```python
from build123d import *

# Parameters (mm, degrees)
ESBO_O1_R                = 2.5
ESBO_O1_W                = 20
ESBO_O1_H                = 40
RESSALTO_EXTRUS_O1_DEPTH = 20
RESSALTO_EXTRUS_O2_DEPTH = 20


with BuildPart() as part:
    # Esboço1 → Ressalto-extrusão1 (new body)
    with BuildSketch(Plane.XY):
        Polygon((2.323964608, -15.698616601), (-17.676035392, -15.698616601), (-21.676035392, -15.698616601), (-21.676035392, 34.301383399), (-21.676035392, 44.301383399), (6.323964608, 44.301383399), (6.323964608, 34.301383399), (6.323964608, -15.698616601), align=None)
        with Locations((-12.176035392, -9.998616601)):
            Circle(ESBO_O1_R, mode=Mode.SUBTRACT)
        with Locations((-3.176035392, -9.998616601)):
            Circle(ESBO_O1_R, mode=Mode.SUBTRACT)
        with Locations((-12.176035392, 38.601383399)):
            Circle(ESBO_O1_R, mode=Mode.SUBTRACT)
        with Locations((-3.176035392, 38.601383399)):
            Circle(ESBO_O1_R, mode=Mode.SUBTRACT)
        with Locations((-7.676035392, 14.301383399)):
            Rectangle(ESBO_O1_W, ESBO_O1_H, mode=Mode.SUBTRACT)
    extrude(amount=RESSALTO_EXTRUS_O1_DEPTH)

    # Esboço2 → Ressalto-extrusão2 (add)
    with BuildSketch(Plane(origin=(0, 0, 0), x_dir=(-1, 0, 0), z_dir=(0, 0, -1))):
        Polygon((-6.323964608, 44.301383399), (-6.323964608, -15.698616601), (-11.323964608, -15.698616601), (-11.323964608, 96.069751334), (-6.323964608, 96.069751334), align=None)
    extrude(amount=-RESSALTO_EXTRUS_O2_DEPTH)


solid = part.part
```
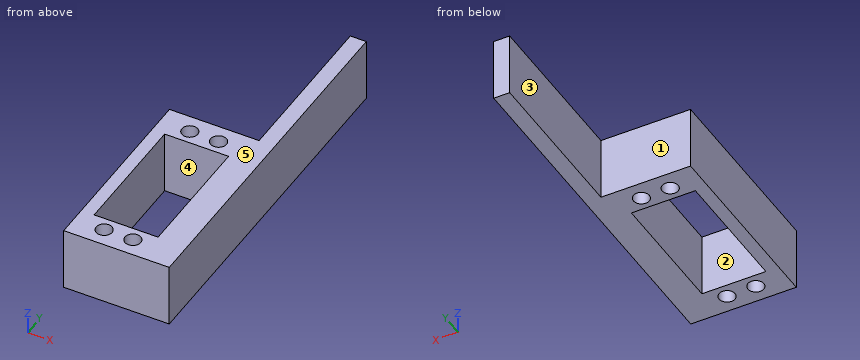
The listing builds one solid part. Answer for the finished solid, in the listing's coordinates (mm). Face numbers are marked on the shaded views. A direction names the side the tool comes from. Coordinates: 2 decimals unless noted, no trailing zeros. Loops run counter-clockwise (first coordinate to the right, second up) from the corner with the lowest first, then second, coordinate; pieces in that order, holes last. Notation, with made-up numbers: (-9.5, 38.25) - (44.5, 38.25) arc R31 cw to (44.5, 74.25) - close; hole circle Ø6 at (84.25, 74.5). An arc over 180 degrees is marked (long way). Write item = value, one per line.
1) Determine the mould class of the marked faces 1, 2 and 3 for opening direction Y: pulls with the +Y half, pulls with the -Y half, needs draft (parallel to the pull), parting line crosses it, or undercut.
Responses:
face_1 = pulls with the +Y half
face_2 = undercut
face_3 = needs draft
2) Which of the six approach directions +Z, -Z, +X, -X, +Y, -Y give full straight-line access (tool end or side, diameter ignored) to the marked faces 4 and 5?
Responses:
face_4 = +Z, -Z
face_5 = +Z, +X, -X, +Y, -Y
3) Find the intervals of material crossed by line 1 along X through (y, z) = (4.5, 18.25); line 2 along Y through (x, z) = (-6.5, 17.25); line 3 along Y through (x, z) = (-11, 19), in increasing order.
Responses:
line_1 = -21.68 to -17.68, 2.32 to 11.32
line_2 = -15.7 to -5.7, 34.3 to 44.3
line_3 = -15.7 to -12.2, -7.79 to -5.7, 34.3 to 36.4, 40.81 to 44.3
4) Section D-D (x = 4) is taken. Determine the outline of the cut face in (y, z).
Responses:
outline = (-15.7, 0) - (44.3, 0) - (44.3, 20) - (-15.7, 20) - close
5) Each of these flat-tipped pins is pushed along its axis until it touches: P1, Ø8, axis at x = -8, z = 4, coming from the +Y side; P2, Ø3, axis at x = -12.18, y = 38.6, coming from the -Z side; P3, Ø2, axis at y = 68.5, z = 3.5, coming from the -X side. Where does it stop, or does it pass through?
Responses:
P1 = 44.3
P2 = through
P3 = 6.32
6) Section C-C (z = 1.5) is taken. Determine the outline of the cut face in (x, y).
Responses:
outline = (-21.68, -15.7) - (11.32, -15.7) - (11.32, 96.07) - (6.32, 96.07) - (6.32, 44.3) - (-21.68, 44.3) - close; hole (-17.68, -5.7) - (2.32, -5.7) - (2.32, 34.3) - (-17.68, 34.3) - close; hole circle Ø5 at (-12.18, -10); hole circle Ø5 at (-12.18, 38.6); hole circle Ø5 at (-3.18, -10); hole circle Ø5 at (-3.18, 38.6)
7) Section B-B (x = -11) is taken. Determine the outline of the cut face in (y, z), plus the area to 3 significant figures.
Responses:
outline = (-15.7, 0) - (-12.2, 0) - (-12.2, 20) - (-15.7, 20) - close; (-7.79, 0) - (-5.7, 0) - (-5.7, 20) - (-7.79, 20) - close; (34.3, 0) - (36.4, 0) - (36.4, 20) - (34.3, 20) - close; (40.81, 0) - (44.3, 0) - (44.3, 20) - (40.81, 20) - close
area = 224 mm^2
8) Section A-A (y = 20) is taken. Determine the outline of the cut face in (x, z), plus the area to 3 significant figures.
Responses:
outline = (-21.68, 0) - (-17.68, 0) - (-17.68, 20) - (-21.68, 20) - close; (2.32, 0) - (11.32, 0) - (11.32, 20) - (2.32, 20) - close
area = 260 mm^2
